```python
from build123d import *

# Parameters (mm, degrees)
SKETCH1_W           = 13.9
SKETCH1_H           = 4.8
BOSS_EXTRUDE1_DEPTH = 6
SKETCH2_W           = 12.6
SKETCH2_H           = 3.500000001
CUT_EXTRUDE1_DEPTH  = 4.25
SKETCH4_W           = 1
SKETCH4_H           = 4.8
BOSS_EXTRUDE2_DEPTH = 1.6
SKETCH5_W           = 0.8
SKETCH5_H           = 1.9
CUT_EXTRUDE3_DEPTH  = 16.328731193
SKETCH3_W           = 1
SKETCH3_H           = 4.000000001
SKETCH3_W_2         = 7.6
SKETCH3_H_2         = 4.25
CUT_EXTRUDE2_DEPTH  = 0.599999999
CUT_EXTRUDE4_START  = -6.3
CUT_EXTRUDE4_DEPTH  = 12.6
BOSS_EXTRUDE3_START = 5
BOSS_EXTRUDE3_DEPTH = 0.25
LPATTERN1_COUNT     = 6
LPATTERN1_PITCH     = 2


with BuildPart() as part:
    # Sketch1 → Boss-Extrude1 (new body)
    with BuildSketch(Plane(origin=(0, 0, 0), x_dir=(1, 0, 0), z_dir=(0, 1, 0))):
        Rectangle(SKETCH1_W, SKETCH1_H)
    extrude(amount=BOSS_EXTRUDE1_DEPTH)

    # Sketch2 → Cut-Extrude1 (cut)
    with BuildSketch(Plane(origin=(0, 6, 0), x_dir=(1, 0, 0), z_dir=(0, 1, 0))):
        with Locations((0, 0.05)):
            Rectangle(SKETCH2_W, SKETCH2_H)
    extrude(amount=-CUT_EXTRUDE1_DEPTH, mode=Mode.SUBTRACT)

    # Sketch4 → Boss-Extrude2 (add)
    with BuildSketch(Plane.XZ):
        with Locations((-6.45, 0)):
            Rectangle(SKETCH4_W, SKETCH4_H)
        with Locations((6.45, 0)):
            Rectangle(SKETCH4_W, SKETCH4_H)
    extrude(amount=BOSS_EXTRUDE2_DEPTH)

    # Sketch5 → Cut-Extrude3 (cut, through all)
    with BuildSketch(Plane.ZY.offset(6.95)):
        Polygon((-2.4, 0), (-1.3, 0), (-0.376239569, -1.6), (-2.4, -1.6), align=None)
        with Locations((-0.55, 5.05)):
            Rectangle(SKETCH5_W, SKETCH5_H)
    extrude(amount=-CUT_EXTRUDE3_DEPTH, mode=Mode.SUBTRACT)

    # Sketch3 → Cut-Extrude2 (cut)
    with BuildSketch(Plane(origin=(0, 0, -2.4), x_dir=(-1, 0, 0), z_dir=(0, 0, -1))):
        with Locations((-5.8, 2.000000001)):
            Rectangle(SKETCH3_W, SKETCH3_H)
        with Locations((0, 3.875)):
            Rectangle(SKETCH3_W_2, SKETCH3_H_2)
        with Locations((5.8, 2.000000001)):
            Rectangle(SKETCH3_W, SKETCH3_H)
    extrude(amount=-CUT_EXTRUDE2_DEPTH, mode=Mode.SUBTRACT)

    # Sketch6 → Cut-Extrude4 (cut)
    with BuildSketch(Plane(origin=(0, 0, 0), x_dir=(0, 0, -1), z_dir=(1, 0, 0)).offset(CUT_EXTRUDE4_START)):
        Polygon((0.15, 1.75), (-1.7, 1.75), (-1.7, 1.15), (-0.45, 1.15), align=None)
    extrude(amount=CUT_EXTRUDE4_DEPTH, mode=Mode.SUBTRACT)


with BuildPart() as body_2:
    # Sketch7 → Boss-Extrude3 (new, symmetric)
    with BuildSketch(Plane(origin=(0, 0, 0), x_dir=(0, 0, -1), z_dir=(1, 0, 0)).offset(BOSS_EXTRUDE3_START)):
        with BuildLine():
            Line((0.45, 5.05), (0.95, 5.05))
            Line((0.95, 5.05), (0.95, 0))
            ThreePointArc((0.95, 0), (0.803553391, -0.353553391), (0.45, -0.5))
            Line((0.45, -0.5), (-4.05, -0.5))
            Line((-4.05, -0.5), (-4.05, 0))
            Line((-4.05, 0), (0.45, 0))
            Line((0.45, 0), (0.45, 5.05))
        make_face()
    extrude(amount=BOSS_EXTRUDE3_DEPTH, both=True)


with BuildPart() as lpattern1_1:
    # LPattern1: pattern copy
    add(body_2.part.moved(Location(Vector(-1, 0, 0) * (1 * LPATTERN1_PITCH))))


with BuildPart() as lpattern1_2:
    # LPattern1: pattern copy
    add(body_2.part.moved(Location(Vector(-1, 0, 0) * (2 * LPATTERN1_PITCH))))


with BuildPart() as lpattern1_3:
    # LPattern1: pattern copy
    add(body_2.part.moved(Location(Vector(-1, 0, 0) * (3 * LPATTERN1_PITCH))))


with BuildPart() as lpattern1_4:
    # LPattern1: pattern copy
    add(body_2.part.moved(Location(Vector(-1, 0, 0) * (4 * LPATTERN1_PITCH))))


with BuildPart() as lpattern1_5:
    # LPattern1: pattern copy
    add(body_2.part.moved(Location(Vector(-1, 0, 0) * (5 * LPATTERN1_PITCH))))


with BuildPart() as lpattern1_4_1:
    add(lpattern1_4.part)

    # Combine1: union body 2, LPattern1_2, LPattern1_5, part, LPattern1_3, LPattern1_1
    add(body_2.part)
    add(lpattern1_2.part)
    add(lpattern1_5.part)
    add(part.part)
    add(lpattern1_3.part)
    add(lpattern1_1.part)


solid = lpattern1_4_1.part
```
Build history of the part. All positions in model axes, mm. A direction names the side the tool comes from. Round coordinates to 2 decimals unless told otherwise and drop trailing zeros. Loops run counter-clockwise (first coordinate to the right, second up) from the corner with the lowest first, then second, coordinate; pieces in that order, holes last.
Item 1: Saw through at B-B (x = 3). List the corners of the cut face in (y, z), then the cut area to 3 significant figures.
Item 2: Saw through at C-C (y = 0.5). List the corners of the cut face in (x, z), then the cut area to 3 significant figures.
Item 3: Pin check, flat tips, straight feed: P1, Ø1, axis at x = -2.5, z = 3.5, coming from the -Y side; P2, Ø0.8, axis at x = 5, y = 4.5, coming from the +Z side. Stop position of each tip, or through.
Item 4: Drill centre lines: line 1 along Z through (x, y) = (5, 4.25); line 2 along X through (y, z) = (2.5, -1.5); line 3 along Z through (x, y) = (-1, 3.75). Where is each one in solid material? Low to high.
Item 5: Which spindle directions (+Z, -Z, +X, -X, +Y, -Y) get a long thin tool onto all of the face, cutting with end or side? Do faces 4 (the face through (5.95, -1, 1)), 5 (the face through (-6, 1, -1.8)), 6 (the face through (5, 4, -1.8)). Say none if no direction does.
Item 6: Saw through at A-A (z = 3.5). List the corners of the cut face in (x, y).
Item 7: Two-plate mould, pull along X, no slides. Class faces 1 (the face through (6.95, 2, 0)), 2 (the face through (0, 3, 2.4)), 3 (the face through (0, 0, 0)): released by +X, released by -X, zero draft, split by the parting line, or undercut.
Worked answers:
1. outline: (-0.5, -0.45) arc R0.5 ccw to (0, -0.95) - (0, -2.4) - (1.75, -2.4) - (1.75, -0.95) - (5.05, -0.95) - (5.05, -0.45) - (1.75, -0.45) - (1.75, -0.15) - (1.15, 0.45) - (1.15, 1.7) - (6, 1.7) - (6, 2.4) - (0, 2.4) - (0, 4.05) - (-0.5, 4.05) - close
1. area: 14.5 mm2
2. outline: (-6.95, -2.4) - (-6.3, -2.4) - (-6.3, -1.8) - (-5.3, -1.8) - (-5.3, -2.4) - (5.3, -2.4) - (5.3, -1.8) - (6.3, -1.8) - (6.3, -2.4) - (6.95, -2.4) - (6.95, 2.4) - (-6.95, 2.4) - close
2. area: 65.5 mm2
3. P1: stops at y = -0.5
3. P2: stops at z = 2.4
4. line 1: z = -2.4 to -1.8, -0.95 to -0.45, 1.7 to 2.4
4. line 2: x = -6.95 to -6.3, 6.3 to 6.95
4. line 3: z = -0.95 to -0.45, 1.7 to 2.4
5. face 4: +Z, -Z, -Y
5. face 5: -Z, -Y
5. face 6: +Y
6. outline: (-5.25, -0.5) - (-4.75, -0.5) - (-4.75, 0) - (-5.25, 0) - close; (-3.25, -0.5) - (-2.75, -0.5) - (-2.75, 0) - (-3.25, 0) - close; (-1.25, -0.5) - (-0.75, -0.5) - (-0.75, 0) - (-1.25, 0) - close; (0.75, -0.5) - (1.25, -0.5) - (1.25, 0) - (0.75, 0) - close; (2.75, -0.5) - (3.25, -0.5) - (3.25, 0) - (2.75, 0) - close; (4.75, -0.5) - (5.25, -0.5) - (5.25, 0) - (4.75, 0) - close
7. face 1: released by +X
7. face 2: zero draft
7. face 3: undercut
